Autodesk Fusion 360 part; units mm, degrees
sketch "Sketch1" plane through (0, 0, 0) normal (0, 0, 1) x (1, 0, 0)
  line L0 (25, -3) -> (25, 3)
  circle A0 centre (0, 0) radius 0.5
  line L1 (25, 0) -> (21, 0)
  line L2 (21, 0) -> (21, -2)
  line L3 (21, -2) -> (25, -2)
  line L4 (25, -2) -> (25, 0)
  line L5 (25, 0) -> (11, 0)
  line L6 (25, 4.5) -> (25, 0)
  line L7 (11, 0) -> (25, 0)
  line L8 (25, 0) -> (25, -4.5)
  line L9 (25, 0) -> (21, 0)
  line L10 (21, 0) -> (21, 2)
  line L11 (21, 2) -> (25, 2)
  line L12 (25, 2) -> (25, 0)
  line L13 (25, -2) -> (21, -2)
  line L14 (25, -4.5) -> (25, -2)
  line L15 (25, 2) -> (21, 2)
  line L16 (25, 4.5) -> (25, 2)
  line L17 (0, 3) -> (11, 6)
  line L18 (0, -3) -> (11, -6)
  line L19 (11, -6) -> (14, -6)
  line L20 (14, -6) -> (25, -4.5)
  line L21 (11, 6) -> (14, 6)
  line L22 (14, 6) -> (25, 4.5)
  arc A1 (0, 3) -> (0, -3) centre (0, 0) ccw
  dimension "d1" = 6
  dimension "d3" = 1
extrude "Extrude1" add sketch "Sketch1" along normal blind 4 contours L0 L2 L3 L6 L8 L10 L11 L13 L14 L15 L16 L17 L18 L19 L20 L21 L22 A1
fillet "Fillet1" radius 0.5 1 edges at (25, -4.5, 2)
fillet "Fillet2" radius 0.5 1 edges at (25, 4.5, 2)
fillet "Fillet3" radius 0.5 1 edges at (14, 6, 2)
fillet "Fillet4" radius 0.5 1 edges at (11, 6, 2)
fillet "Fillet5" radius 0.5 1 edges at (14, -6, 2)
fillet "Fillet6" radius 0.5 1 edges at (11, -6, 2)
sketch "Sketch2" plane through (0, 0, 0) normal (0, 0, 1) x (1, 0, 0)
sketch "Sketch3" plane through (0, 0, 0) normal (0, 1, 0) x (1, 0, 0)
sketch "Sketch6" plane through (0, 0, 0) normal (0, 0, -1) x (1, 0, 0)
  circle A0 centre (0, 0) radius 0.5
  arc A1 (11.067, 6) -> (10.9354, 5.9824) centre (11.067, 5.5) ccw
  line L0 (10.9354, 5.9824) -> (0, 3)
  arc A2 (0, 3) -> (0, -3) centre (0, 0) ccw
  line L1 (0, -3) -> (10.9354, -5.9824)
  arc A3 (10.9354, -5.9824) -> (11.067, -6) centre (11.067, -5.5) ccw
  line L2 (11.067, -6) -> (13.9661, -6)
  arc A4 (13.9661, -6) -> (14.0336, -5.9954) centre (13.9661, -5.5) ccw
  line L3 (14.0336, -5.9954) -> (24.5676, -4.559)
  arc A5 (24.5676, -4.559) -> (25, -4.0636) centre (24.5, -4.0636) ccw
  line L4 (25, -4.0636) -> (25, -2)
  line L5 (25, -2) -> (21, -2)
  line L6 (21, -2) -> (21, 2)
  line L7 (21, 2) -> (25, 2)
  line L8 (25, 2) -> (25, 4.0636)
  arc A6 (25, 4.0636) -> (24.5676, 4.559) centre (24.5, 4.0636) ccw
  line L9 (24.5676, 4.559) -> (14.0336, 5.9954)
  arc A7 (14.0336, 5.9954) -> (13.9661, 6) centre (13.9661, 5.5) ccw
  line L10 (13.9661, 6) -> (11.067, 6)
  line L11 (11.067, 6) -> (11.067, -6)
  dimension "d22" = 21
sketch "Sketch7" plane through (0, 0, 4) normal (0, 0, 1) x (-1, 0, 0)
  arc A0 (-10.9354, 5.9824) -> (-11.067, 6) centre (-11.067, 5.5) ccw
  line L0 (-11.067, 6) -> (-13.9661, 6)
  arc A1 (-13.9661, 6) -> (-14.0336, 5.9954) centre (-13.9661, 5.5) ccw
  line L1 (-14.0336, 5.9954) -> (-24.5676, 4.559)
  arc A2 (-24.5676, 4.559) -> (-25, 4.0636) centre (-24.5, 4.0636) ccw
  line L2 (-25, 4.0636) -> (-25, 2)
  line L3 (-25, 2) -> (-21, 2)
  line L4 (-21, 2) -> (-21, -2)
  line L5 (-21, -2) -> (-25, -2)
  line L6 (-25, -2) -> (-25, -4.0636)
  arc A3 (-25, -4.0636) -> (-24.5676, -4.559) centre (-24.5, -4.0636) ccw
  line L7 (-24.5676, -4.559) -> (-14.0336, -5.9954)
  arc A4 (-14.0336, -5.9954) -> (-13.9661, -6) centre (-13.9661, -5.5) ccw
  line L8 (-13.9661, -6) -> (-11.067, -6)
  arc A5 (-11.067, -6) -> (-10.9354, -5.9824) centre (-11.067, -5.5) ccw
  line L9 (-10.9354, -5.9824) -> (0, -3)
  arc A6 (0, -3) -> (0, 3) centre (0, 0) ccw
  line L10 (0, 3) -> (-10.9354, 5.9824)
  circle A7 centre (0, 0) radius 0.5
  line L11 (0, 0) -> (-12.5, 0)
  line L12 (-12.5, 0) -> (-12.5, -1.5)
  line L13 (-12.5, 0) -> (-12.5, 1.5)
  circle A8 centre (-12.5, -1.5) radius 0.5
  circle A9 centre (-12.5, 1.5) radius 0.5
  dimension "d23" = 12.5
  dimension "d24" = 1
  dimension "d25" = 1
hole "Hole1" at (12.5, 1.5, 4) direction (0, 0, -1) diameter 1 depth 2 tip angle 118
hole "Hole2" at (12.5, -1.5, 4) direction (0, 0, -1) diameter 1 depth 2 tip angle 118
ref_plane "WorkPlane1" through (0, 0, 12) normal (0, 0, 1) x (1, 0, 0)
equation "d25 = mm"
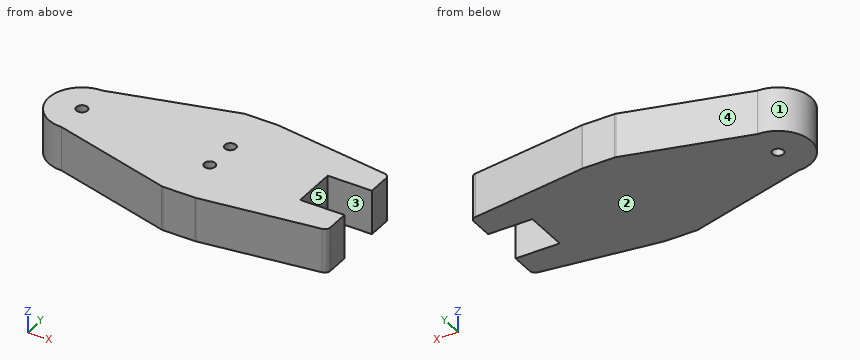
Build history of the part. All positions in model axes, mm. Face numbers are marked on the shaded views. A direction names the side the tool comes from. Coordinates: 2 decimals unless noted, no trailing zeros. Write each loop counter-clockwise with the first axis right and the second up, starting at its lowest first coordinate (ties: lowest second). Pieces come first, ordered by that corner, then holes.
1. 3-axis set-ups, long thin cutter, end or side, ignore diameter. For the marked faces 4 and 5: which of +Z, -Z, +X, -X, +Y, -Y reach the whole face in a straight line?
Answer block:
face 4: +Z, -Z, -X, +Y
face 5: +Z, -Z, +X
2. Drill centre lines: probe 1 along Y at (x, z) = (12.5, 3.3); probe 2 along X at (y, z) = (-1.75, 3.2); probe 3 along Y at (x, z) = (14, 2.4). Where is each one in solid material? Low to high.
Answer block:
probe 1: y = -6 to -2, -1 to 1, 2 to 6
probe 2: x = -2.44 to 12.07, 12.93 to 21
probe 3: y = -6 to 6
3. Band-saw the part on A-A, the plane y = 0. Give the cut face in (x, z).
Answer block:
outline: (-3, 0) - (-0.5, 0) - (-0.5, 4) - (-3, 4) - close; (0.5, 0) - (21, 0) - (21, 4) - (0.5, 4) - close
4. Band-saw the part on C-C, the plane z = 3.3. Give the cut face in (x, y), and give its area (3 significant figures).
Answer block:
outline: (0, -3) - (10.94, -5.98) arc R0.5 ccw to (11.07, -6) - (13.97, -6) arc R0.5 ccw to (14.03, -6) - (24.57, -4.56) arc R0.5 ccw to (25, -4.06) - (25, -2) - (21, -2) - (21, 2) - (25, 2) - (25, 4.06) arc R0.5 ccw to (24.57, 4.56) - (14.03, 6) arc R0.5 ccw to (13.97, 6) - (11.07, 6) arc R0.5 ccw to (10.94, 5.98) - (0, 3) arc R3 ccw to start; hole circle Ø1 at (0, 0); hole circle Ø1 at (12.5, -1.5); hole circle Ø1 at (12.5, 1.5)
area: 246 mm2
5. Band-saw the part on B-B, the plane z = 0.9. Give the cut face in (x, y).
Answer block:
outline: (0, -3) - (10.94, -5.98) arc R0.5 ccw to (11.07, -6) - (13.97, -6) arc R0.5 ccw to (14.03, -6) - (24.57, -4.56) arc R0.5 ccw to (25, -4.06) - (25, -2) - (21, -2) - (21, 2) - (25, 2) - (25, 4.06) arc R0.5 ccw to (24.57, 4.56) - (14.03, 6) arc R0.5 ccw to (13.97, 6) - (11.07, 6) arc R0.5 ccw to (10.94, 5.98) - (0, 3) arc R3 ccw to start; hole circle Ø1 at (0, 0)
6. Band-saw the part on D-D, the plane x = 4.25. Give the cut face in (y, z).
Answer block:
outline: (-4.16, 0) - (4.16, 0) - (4.16, 4) - (-4.16, 4) - close
7. Drop flat-ended pins along their axis: pin 1 (1 mm diameter, centred on x = 7, z = 2.5, fed in from +Y); pin 2 (2 mm diameter, centred on x = 4, z = 2, fed in from -Y); pin 3 (2 mm diameter, centred on x = 24, z = 3, fed in from -Y); pin 4 (1.5 mm diameter, centred on y = -0.5, z = 1, fed in from -X). Give the stop position or say it passes through.
Answer block:
pin 1: stops at y = 5.05
pin 2: stops at y = -4.36
pin 3: stops at y = -4.77
pin 4: stops at x = -3
8. Pull direction Y, two halves, no side cores. Call the marked faces 1, 2 and 3: released by +Y, released by -Y, zero draft, split by the parting line, or undercut.
Answer block:
face 1: split by the parting line
face 2: zero draft
face 3: undercut
